Verification items for the finished model (mm, model axes). A direction names the side the tool comes from. Round coordinates to 2 decimals unless told otherwise and drop trailing zeros. Write each loop counter-clockwise with the first axis right and the second up, starting at its lowest first coordinate (ties: lowest second). Pieces come first, ordered by that corner, then holes.
from build123d import *

# Parameters (mm, degrees)
EXTRUDE_1_DEPTH     = 28.5
SKETCH_2_R          = 2.525
CUT_EXTRUDE_1_DEPTH = 28.5
HOLE_WIZARD_M4_1_D  = 3.3
FILLET_1_R          = 2
FILLET_2_R          = 1


with BuildPart() as part:
    # 草图1 → 凸台-拉伸1 (new body)
    with BuildSketch(Plane.XY):
        Polygon((0, 0), (-10, 0), (-10, 5), (5, 5), (5, -18), (0, -18), align=None)
    extrude(amount=EXTRUDE_1_DEPTH)

    # 草图2 → 切除-拉伸1 (cut)
    with BuildSketch(Plane(origin=(0, 5, 0), x_dir=(1, 0, 0), z_dir=(0, 1, 0))):
        with Locations((-5.5, -4.15)):
            Circle(SKETCH_2_R)
        with Locations((-5.5, -20.15)):
            Circle(SKETCH_2_R)
    extrude(amount=-CUT_EXTRUDE_1_DEPTH, mode=Mode.SUBTRACT)

    # M4 螺纹孔1 (through all)
    with Locations(Plane(origin=(0, -5, 10.5), x_dir=(0, -1, 0), z_dir=(-1, 0, 0))):
        with Locations((0, 0), (10, 0), (10, 11), (0, 11)):
            Hole(HOLE_WIZARD_M4_1_D / 2)

    # 圆角1
    fillet_1_edges = [part.edges().sort_by_distance(p)[0] for p in [
        (-10, 2.5, 28.5),
        (-10, 2.5, 0),
    ]]
    fillet(fillet_1_edges, radius=FILLET_1_R)

    # 圆角2
    fillet_2_edges = [part.edges().sort_by_distance(p)[0] for p in [
        (0, 0, 14.25),
        (5, 5, 14.25),
        (5, -18, 14.25),
    ]]
    fillet(fillet_2_edges, radius=FILLET_2_R)


solid = part.part
Q1. Release check for a two-part mould opening along Y. For faces 1 (the flat face through (-10, 2, 14)), 2 (the cylindrical face through (-0.301, -0.285, 14.45)), 3 (the flat face through (-3, 5, 14)), 4 (the cylindrical face through (2.535, -5.215, 23.136)) record: released by +Y, released by -Y, zero draft, split by the parting line, or undercut.
Recorded:
face 1: zero draft
face 2: released by -Y
face 3: released by +Y
face 4: undercut
Q2. Tool access check on faces 5 (the cylindrical face through (4.699, 4.715, 14.45)), 6 (the flat face through (-5, 0, 14)). Record the directions out of +Z, -Z, +X, -X, +Y, -Y that give a thin tool (end or side, any length) a straight path to the whole face; none if there is none.
Recorded:
face 5: +Z, -Z, +X, +Y
face 6: +Z, -Z, -X, -Y
Q3. Sectioned sample at B-B (y = -15). Enter the section's corners in (x, z).
Recorded:
outline: (0, 0) - (5, 0) - (5, 8.85) - (0, 8.85) - close; (0, 12.15) - (5, 12.15) - (5, 19.85) - (0, 19.85) - close; (0, 23.15) - (5, 23.15) - (5, 28.5) - (0, 28.5) - close
Q4. Sectioned sample at C-C (z = 10.5). Enter the section's corners in (x, y).
Recorded:
outline: (-10, 0) - (-1, 0) arc R1 cw to (0, -1) - (0, -3.35) - (5, -3.35) - (5, 4) arc R1 ccw to (4, 5) - (-10, 5) - close; (0, -18) - (4, -18) arc R1 ccw to (5, -17) - (5, -16.65) - (0, -16.65) - close; (0, -13.35) - (5, -13.35) - (5, -6.65) - (0, -6.65) - close
Q5. Sectioned sample at A-A (x = -5.5). Enter the section's corners in (y, z) (3 decimals), plus the area to 3 significant figures.
Recorded:
outline: (0, 0) - (5, 0) - (5, 1.625) - (0, 1.625) - close; (0, 6.675) - (5, 6.675) - (5, 17.625) - (0, 17.625) - close; (0, 22.675) - (5, 22.675) - (5, 28.5) - (0, 28.5) - close
area: 92.0 mm2
Q6. Sectioned sample at D-D (y = 2.75). Enter the section's corners in (x, z) (3 decimals), plus the area to 3 significant figures.
Recorded:
outline: (-10, 2) arc R2 ccw to (-8, 0) - (5, 0) - (5, 28.5) - (-8, 28.5) arc R2 ccw to (-10, 26.5) - close; hole circle Ø5.05 at (-5.5, 4.15); hole circle Ø5.05 at (-5.5, 20.15)
area: 386 mm2
Q7. Material ranges on line 1 along Z through (x, y) = (-5.5, 3.3) (3 decimals); line 2 along Z through (x, y) = (3, -5); line 3 along X through (y, z) = (3.55, 4.15) (3 decimals), recorded low to high.
Recorded:
line 1: z = 0 to 1.625, 6.675 to 17.625, 22.675 to 28.5
line 2: z = 0 to 8.85, 12.15 to 19.85, 23.15 to 28.5
line 3: x = -10 to -8.025, -2.975 to 5
Q8. Depth check by flat-ended pin: P1, Ø2.5, axis at y = -5, z = 10.5, coming from the +X side; P2, Ø2, axis at y = -13.5, z = 25, coming from the -X side; P3, Ø1.5, axis at x = -6, z = 12, coming from the -Y side. Enter the tip coordinate at first touch or a pass-through.
Recorded:
P1: passes through
P2: stops at x = 0
P3: stops at y = 0
